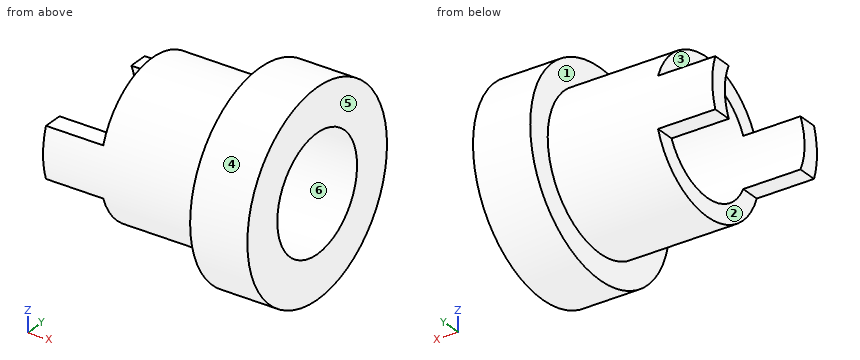
```python
from build123d import *

# Parameters (mm, degrees)
SKETCH2_W          = 3.5
SKETCH2_H          = 9.899494936
CUT_EXTRUDE1_DEPTH = 4


with BuildPart() as part:
    # Sketch1 → Revolve1 (revolve)
    with BuildSketch(Plane(origin=(0, 0, 0), x_dir=(1, 0, 0), z_dir=(0, 1, 0))):
        Polygon((0, 4), (0, 7), (-4, 7), (-4, 5.25), (-15.5, 5.25), (-15.5, 4), align=None)
    revolve(axis=Axis((-5.134665776, 0, 0), (1, 0, 0)))

    # Sketch2 → Cut-Extrude1 (cut)
    with BuildSketch(Plane.ZY.offset(15.5)):
        with Locations((-3.5, 0)):
            Rectangle(SKETCH2_W, SKETCH2_H)
        with Locations((3.5, 0)):
            Rectangle(SKETCH2_W, SKETCH2_H)
    extrude(amount=-CUT_EXTRUDE1_DEPTH, mode=Mode.SUBTRACT)


solid = part.part
```
CAD build for the part. Positions are in the model's coordinates, mm. Face numbers are marked on the shaded views. A direction names the side the tool comes from. Round coordinates to 2 decimals unless told otherwise and drop trailing zeros. Loops run counter-clockwise (first coordinate to the right, second up) from the corner with the lowest first, then second, coordinate; pieces in that order, holes last. Notation, with made-up numbers: (-19.5, -36.75) - (13.5, -36.75) arc R14 ccw to (13.5, -31.75) - close; hole circle Ø9 at (-39, 57). An arc over 180 degrees is marked (long way). Return JSON: item names as keys, results as strings. Group by question number.
Q1. Band-saw the part on B-B on y = 0. Give the cut face in (x, z).
Q2. Band-saw the part on C-C on z = 0. Give the cut face in (x, y), plus the area to 4 significant figures.
Q3. Drill centre lines: line 1 along Z through (x, y) = (-6.75, 0); line 2 along X through (y, z) = (-2, 3.75). Where is each one in solid material? Low to high. Write a range as [from, to].
Q4. Band-saw the part on D-D on x = -8.75. Give the cut face in (y, z).
Q5. Band-saw the part on A-A on x = -12.5. Give the cut face in (y, z), plus the area to 3 significant figures.
Q6. Two-plate mould, pull along Y, no slides. Class the marked faces 4, 5 and 6: +Y half, -Y half, draft (parallel to the pull), parting line (faces both ways), or undercut.
Q7. Flat gauge pins, fed straight in: pin 1 Ø4 at (x, z) = (-9.5, 4.5) entering from -Y; pin 2 Ø1.8 at (y, z) = (1.5, -3.5) entering from -X; pin 3 Ø1.5 at (x, y) = (-11, 1.5) entering from -Z. Where does each tip first touch, or does it go through?
Q8. Tool access for the marked faces 1, 2 and 3: list every direction of +Z, -Z, +X, -X, +Y, -Y with a clear straight run to the whole face (end or side of a thin tool).
Solutions:
{
 "1": {"outline": "(-11.5, -5.25) - (-4, -5.25) - (-4, -7) - (0, -7) - (0, -4) - (-11.5, -4) - close; (-11.5, 4) - (0, 4) - (0, 7) - (-4, 7) - (-4, 5.25) - (-11.5, 5.25) - close"},
 "2": {"outline": "(-15.5, -5.25) - (-4, -5.25) - (-4, -7) - (0, -7) - (0, -4) - (-15.5, -4) - close; (-15.5, 4) - (0, 4) - (0, 7) - (-4, 7) - (-4, 5.25) - (-15.5, 5.25) - close", "area": "52.75 mm^2"},
 "3": {"line 1": "z = [-5.25, -4], [4, 5.25]", "line 2": "x = [-11.5, 0]"},
 "4": {"outline": "circle Ø10.5 at (0, 0); hole circle Ø8 at (0, 0)"},
 "5": {"outline": "(-4.95, -1.75) - (-3.6, -1.75) arc R4 cw to (-3.6, 1.75) - (-4.95, 1.75) arc R5.25 ccw to start; (3.6, -1.75) - (4.95, -1.75) arc R5.25 ccw to (4.95, 1.75) - (3.6, 1.75) arc R4 cw to start", "area": "8.98 mm^2"},
 "6": {"face 4": "parting line", "face 5": "draft", "face 6": "undercut"},
 "7": {"pin 1": "stops at y = -4.62", "pin 2": "stops at x = -11.5", "pin 3": "stops at z = -5.2"},
 "8": {"face 1": "-X", "face 2": "-Z, -X, +Y, -Y", "face 3": "+Z, -X, +Y, -Y"}
}
